The model under review builds one solid part; all positions refer to its coordinate system, in mm. A direction names the side the tool comes from. Round coordinates to 2 decimals unless told otherwise and drop trailing zeros. Order: outer loops, then holes, each group sorted by start corner. A loop starts at its lowest first (then second) coordinate and runs counter-clockwise, first axis right, second up.
```python
from build123d import *

# Parameters (mm, degrees)
F1_DEPTH = 30
F2_W     = 119.865141
F2_H     = 64.247175
F3_DEPTH = 28
F4_W     = 136.580032
F4_H     = 69.443569
F5_DEPTH = 3


with BuildPart() as f1:
    # F0 (on Top) → F1 (new body)
    with BuildSketch(Plane.XY):
        with BuildLine():
            ThreePointArc((0, -6.35), (-1.859872, -1.859872), (-6.35, 0))
            Line((-6.35, 0), (-126.215141, 0))
            ThreePointArc((-126.215141, 0), (-130.705269, -1.859872), (-132.565141, -6.35))
            Line((-132.565141, -6.35), (-132.565141, -70.597175))
            ThreePointArc((-132.565141, -70.597175), (-130.705269, -75.087303), (-126.215141, -76.947175))
            Line((-126.215141, -76.947175), (-6.35, -76.947175))
            ThreePointArc((-6.35, -76.947175), (-1.859872, -75.087303), (0, -70.597175))
            Line((0, -70.597175), (0, -6.35))
        make_face()
    extrude(amount=F1_DEPTH)

    # F2 (on face) → F3 (cut)
    with BuildSketch(Plane.XY.offset(30)):
        with Locations((-66.28257, -38.473587)):
            Rectangle(F2_W, F2_H)
    extrude(amount=-F3_DEPTH, mode=Mode.SUBTRACT)

    # F4 (on face) → F5 (cut)
    with BuildSketch(Plane.XY.offset(30)):
        with Locations((-60.4819, -38.440659)):
            Rectangle(F4_W, F4_H)
    extrude(amount=-F5_DEPTH, mode=Mode.SUBTRACT)


solid = f1.part
```
(1) To check wall thickness, follow probe 1 along X at (y, z) = (-55, 3.5); probe 2 along Y at (x, z) = (-88, 18.75); probe 3 along Y at (x, z) = (-54, 27.5). State the ranges of each line that lie inside material, in increasing order.
Data:
probe 1: x = -132.57 to -126.22, -6.35 to 0
probe 2: y = -76.95 to -70.6, -6.35 to 0
probe 3: y = -76.95 to -73.16, -3.72 to 0
(2) Insertion check: pin 1 (0.9 mm diameter, centred on y = -53.5, z = 29, fed in from +X). The pin has a flat end and moves straight along its axis. Give the tip position at first contact, or say it passes through.
Data:
pin 1: stops at x = -128.77
(3) For faces 1 (the flat face through (-67, -70.597, 15)), 2 (the flat face through (-66, -73.162, 29)), 3 (the flat face through (-67, -76.947, 15)), list the 3-axis set-ups (+Z, -Z, +X, -X, +Y, -Y) from which the entire face can be reached by the end or side of a thin tool; tool diameter is ignored.
Data:
face 1: +Z
face 2: +Z, +X
face 3: +Z, -Z, +X, -X, -Y
(4) Draft analysis for pull direction Y (two halves, no side actions). For faces 4 (the cylindrical face through (-1.81, -1.91, 14.79)), 5 (the cylindrical face through (-1.91, -75.136, 14.79)), 6 (the flat face through (-128.772, -39, 29)), state which applies: pulls with the +Y half, pulls with the -Y half, needs draft (parallel to the pull), parting line crosses it, or undercut.
Data:
face 4: pulls with the +Y half
face 5: pulls with the -Y half
face 6: undercut
(5) Consider section C-C (x = -56.5). Write out the cut boundary in (y, z).
Data:
outline: (-76.95, 0) - (0, 0) - (0, 30) - (-3.72, 30) - (-3.72, 27) - (-6.35, 27) - (-6.35, 2) - (-70.6, 2) - (-70.6, 27) - (-73.16, 27) - (-73.16, 30) - (-76.95, 30) - close
(6) Consider section B-B (y = -21.5). Write out the cut boundary in (x, z), and give its area (3 significant figures).
Data:
outline: (-132.57, 0) - (0, 0) - (0, 27) - (-6.35, 27) - (-6.35, 2) - (-126.22, 2) - (-126.22, 27) - (-128.77, 27) - (-128.77, 30) - (-132.57, 30) - close
area: 594 mm2
(7) Consider section A-A (z = 22.5). Write out the cut boundary in (x, y), and give its area (3 significant figures).
Data:
outline: (-132.57, -70.6) arc R6.35 ccw to (-126.22, -76.95) - (-6.35, -76.95) arc R6.35 ccw to (0, -70.6) - (0, -6.35) arc R6.35 ccw to (-6.35, 0) - (-126.22, 0) arc R6.35 ccw to (-132.57, -6.35) - close; hole (-126.22, -70.6) - (-6.35, -70.6) - (-6.35, -6.35) - (-126.22, -6.35) - close
area: 2,460 mm2
